from build123d import *

# Parameters (mm, degrees)
SKETCH_1_W      = 1.8
SKETCH_1_H      = 0.8
EXTRUDE_1_DEPTH = 3.5
SKETCH_2_W      = 19.6
SKETCH_2_H      = 1.6
EXTRUDE_2_DEPTH = 1


with BuildPart() as part:
    # 草图1 → 凸台-拉伸1 (new body)
    with BuildSketch(Plane(origin=(0, 0, 0), x_dir=(0, 0, -1), z_dir=(1, 0, 0))):
        Polygon((-8, -0.8), (-8, 0), (-8, 0.8), (-9.8, 0.8), (-9.8, -0.8), align=None)
        with Locations((-7.1, -0.4)):
            Rectangle(SKETCH_1_W, SKETCH_1_H)
        with Locations((-7.1, 0.4)):
            Rectangle(SKETCH_1_W, SKETCH_1_H)
        with Locations((-0.9, 0.4)):
            Rectangle(SKETCH_1_W, SKETCH_1_H)
        with Locations((-0.9, -0.4)):
            Rectangle(SKETCH_1_W, SKETCH_1_H)
        with Locations((0.9, -0.4)):
            Rectangle(SKETCH_1_W, SKETCH_1_H)
        with Locations((0.9, 0.4)):
            Rectangle(SKETCH_1_W, SKETCH_1_H)
        with Locations((7.1, -0.4)):
            Rectangle(SKETCH_1_W, SKETCH_1_H)
        with Locations((7.1, 0.4)):
            Rectangle(SKETCH_1_W, SKETCH_1_H)
        Polygon((8, 0.8), (8, 0), (8, -0.8), (9.8, -0.8), (9.8, 0.8), align=None)
    extrude(amount=EXTRUDE_1_DEPTH)

    # 草图2 → 凸台-拉伸2 (add)
    with BuildSketch(Plane.ZY):
        Rectangle(SKETCH_2_W, SKETCH_2_H)
    extrude(amount=EXTRUDE_2_DEPTH)


solid = part.part
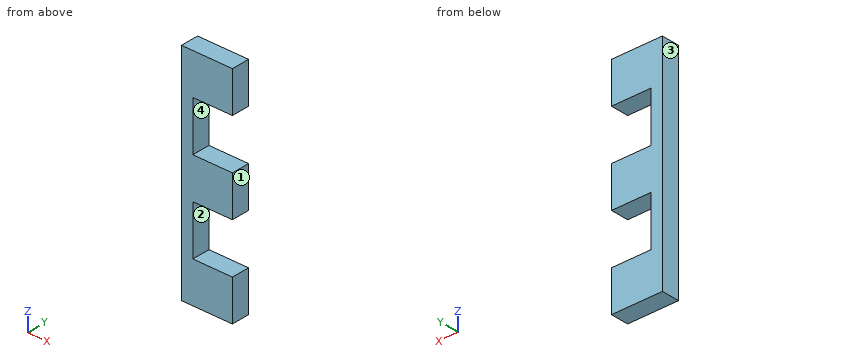
The listing builds one solid part. Answer for the finished solid, in the listing's coordinates (mm). Face numbers are marked on the shaded views. A direction names the side the tool comes from. Coordinates: 2 decimals unless noted, no trailing zeros. Loops run counter-clockwise (first coordinate to the right, second up) from the corner with the lowest first, then second, coordinate; pieces in that order, holes last. Notation, with made-up numbers: (32, -23.75) -> (45, -23.75) arc R18 ccw to (45, 0.25) -> close; hole circle Ø2 at (89, -39). An arc over 180 degrees is marked (long way). Write item = value, one per line. Start each with the question number.
1) The mould has two halves that part along Z. Classify the marked faces 3 and 4: released by +Z, released by -Z, zero draft, split by the parting line, or undercut.
2) Given pin 1 Ø0.8 at (y, z) = (0, 4.5) entering from +X, flat-ended and moving along its own axis, determine where the tip first touches the part or whether it passes through.
3) Straight lines are drawn through the part: line 1 (Z direction, x = 2, y = -0.25); line 2 (X direction, y = -0.3, z = 3.25). For each, find the intervals that lie inside material, in ascending order. Write a range as from..to.
4) A tool of negligible diameter and unlimited length cuts with its end or side. For the marked faces 1 and 2, from which of +Z, -Z, +X, -X, +Y, -Y can it reach the whole face along a straight path? Write none if from no direction.
5) A cutting plane is placed at C-C (z = 5). Give the vertices of the cut face in (x, y).
6) A cutting plane is placed at A-A (x = 1.45). Give the vertices of the cut face in (y, z), then the cut area to 3 significant figures.
7) A cutting plane is placed at B-B (y = -0.25). Give the vertices of the cut face in (x, z), then the cut area to 3 significant figures.
Responses:
q1.face_3 = zero draft
q1.face_4 = undercut
q2.pin_1 = 0
q3.line_1 = -9.8..-6.2, -1.8..1.8, 6.2..9.8
q3.line_2 = -1..0
q4.face_1 = +Z, -Z, +X, +Y, -Y
q4.face_2 = +X, +Y, -Y
q5.outline = (-1, -0.8) -> (0, -0.8) -> (0, 0.8) -> (-1, 0.8) -> close
q6.outline = (-0.8, -9.8) -> (0.8, -9.8) -> (0.8, -6.2) -> (-0.8, -6.2) -> close; (-0.8, -1.8) -> (0.8, -1.8) -> (0.8, 1.8) -> (-0.8, 1.8) -> close; (-0.8, 6.2) -> (0.8, 6.2) -> (0.8, 9.8) -> (-0.8, 9.8) -> close
q6.area = 17.3 mm²
q7.outline = (-1, -9.8) -> (3.5, -9.8) -> (3.5, -6.2) -> (0, -6.2) -> (0, -1.8) -> (3.5, -1.8) -> (3.5, 1.8) -> (0, 1.8) -> (0, 6.2) -> (3.5, 6.2) -> (3.5, 9.8) -> (-1, 9.8) -> close
q7.area = 57.4 mm²
